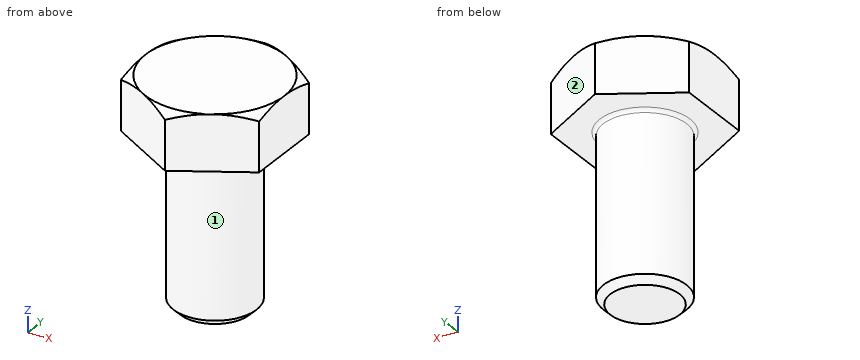
Autodesk Inventor part; units mm, degrees
ref_plane "WorkPlane1" through (0, 0, 0) normal (0, 0, 1) x (1, 0, 0)
ref_plane "MSC_PF1" through (0, 0, 0) normal (1, 0, 0) x (0, 1, 0)
ref_plane "MSC_PT1" through (0, 0, 0) normal (0, 0, -1) x (-1, 0, 0)
ref_plane "WorkPlane1" through (0, 0, 0) normal (0, 0, 1) x (1, 0, 0)
sketch "Sketch1" plane through (0, 0, 0) normal (0, 0, 1) x (1, 0, 0)
  point P0 (0, 0)
sketch "Sketch2" plane through (0, 0, 0) normal (0, 0, 1) x (1, 0, 0)
  line L0 (-5, 2.8868) -> (-5, -2.8868)
  line L1 (0, 5.7734) -> (-5, 2.8868)
  line L2 (5, 2.8868) -> (0, 5.7734)
  line L3 (5, -2.8868) -> (5, 2.8868)
  line L4 (0, -5.7734) -> (5, -2.8868)
  line L5 (-5, -2.8868) -> (0, -5.7734)
  circle A0 centre (0, 0) radius 5 construction
  dimension "d1" = 10
  dimension "d29" = 0
  dimension "d30" = 0
extrude "Extrusion1" add sketch "Sketch2" along normal blind 4
sketch "Sketch3" plane through (0, 0, 0) normal (1, 0, 0) x (0, 1, 0)
  line L0 (5, 4) -> (5.8734, 4)
  line L1 (5.8734, 3.4957) -> (5, 4)
  line L2 (5.8734, 4) -> (5.8734, 3.4957)
  line L3 (0, -0.8) -> (0, 4.8)
  line L4 (5.7734, 0) -> (5.7734, 4)
  dimension "d25" = 0.1
  dimension "d26" = 0
  dimension "d27" = 60
  dimension "d28" = 5
revolve "Revolution1" cut sketch "Sketch3" angle 360 about axis through (0, 0, -10) along (0, 0, 1)
sketch "Sketch4" plane through (0, 0, 0) normal (1, 0, 0) x (0, 1, 0)
  line L0 (0, -12) -> (0, 0)
  line L1 (-3, -12) -> (0, -12)
  line L2 (-3, 0) -> (-3, -12)
  line L3 (0, 0) -> (-3, 0)
  line L4 (0, -12) -> (0, 0)
  line L5 (-3.6, 0) -> (0.6, 0)
  line L6 (0, -14.4) -> (0, 2.4)
  dimension "d18" = 3
  dimension "d20" = 12
  dimension "d33" = 0
  dimension "d34" = 0
revolve "Revolution2" add sketch "Sketch4" angle 360 about axis through (0, 0, -12) along (0, 0, -1)
chamfer "Chamfer1" distance 0.5 angle 45 1 edges at (0, 3, -12)
fillet "Fillet1" radius 0.25 1 edges at (0, 3, 0)
thread "Thread1"
ref_plane "MSC_PF1" through (0, 0, 0) normal (1, 0, 0) x (0, 1, 0)
ref_plane "MSC_PT1" through (0, 0, 0) normal (0, 0, -1) x (-1, 0, 0)
equation "\"d22\" = 0.5 * PTC"
equation "\"d23\" = 0.5 * PTC"
equation "\"d24\" = r"
equation "\"d1\" = ParS"
equation "\"d6\" = ParK"
equation "\"b\" = NLG - 2 * PTC"
equation "\"d28\" = 0.5 * ParS"
equation "\"d18\" = 0.5 * NND"
equation "\"d20\" = NLG"
equation "\"NND\" = 6"
equation "\"NLG\" = 12"
equation "\"PTC\" = 1"
equation "\"ParK\" = 4"
equation "\"ParS\" = 10"
equation "\"msp_es\" = 0.577367 * ParS"
equation "\"r\" = 0.25"
equation "\"THREADDIA\" = NND"
properties part number "ISO 4018 - M6 x 12" material "Steel"
The listing builds one solid part. Answer for the finished solid, in the listing's coordinates (mm). Face numbers are marked on the shaded views. A direction names the side the tool comes from. Round coordinates to 2 decimals unless told otherwise and drop trailing zeros. Loops run counter-clockwise (first coordinate to the right, second up) from the corner with the lowest first, then second, coordinate; pieces in that order, holes last. Notation, with made-up numbers: (-9.75, 69.25) - (41.25, 69.25) arc R20 cw to (41.25, 104.25) - close; hole circle Ø7 at (81.5, 19.5). An arc over 180 degrees is marked (long way). Return JSON: item names as keys, results as strings. Group by question number.
1. Which of the six approach directions +Z, -Z, +X, -X, +Y, -Y give full straight-line access (tool end or side, diameter ignored) to the marked faces 1 and 2?
2. Consider probe 1 along Z at (x, y) = (-1.75, -3.5); probe 2 along X at (y, z) = (-1.5, -10.75); probe 3 along Y at (x, z) = (-2.25, -6.5). Determine where each line is inside the solid, lowest interval first.
3. Each of these flat-tipped pins is pushed along its axis until it touches: P1, Ø1, axis at y = 0.5, z = -6, coming from the -X side; P2, Ø3, axis at x = -3, z = 1.5, coming from the +Y side; P3, Ø6, axis at y = -3, z = -7, coming from the +X side. Where does it stop, or does it pass through?
4. The part is cut by section A-A on z = -4.75. Determine the outline of the cut face in (x, y), then the cut area to 3 significant figures.
Resolved:
{
 "1": {"face 1": "-Z", "face 2": "+Z, -Z, +X, +Y"},
 "2": {"probe 1": "z = 0 to 4", "probe 2": "x = -2.6 to 2.6", "probe 3": "y = -1.98 to 1.98"},
 "3": {"P1": "stops at x = -3", "P2": "stops at y = 4.91", "P3": "stops at x = 3"},
 "4": {"outline": "circle Ø6 at (0, 0)", "area": "28.3 mm²"}
}
